Could you check a few things on this model? Use its own coordinates, in mm. Face numbers are marked on the shaded views. A direction names the side the tool comes from. Give positions to 0.01 mm unless a question says otherwise; leave off trailing zeros. Loops run counter-clockwise (first coordinate to the right, second up) from the corner with the lowest first, then second, coordinate; pieces in that order, holes last. Notation, with made-up numbers: (-14.5, 17.25) - (10.5, 17.25) arc R33 ccw to (10.5, 45.25) - close; hole circle Ø10 at (36.5, 72). An arc over 180 degrees is marked (long way). One line per item, written item: value. Start each with the question number.
Q1. I want a section at A-A (x = -18). Please give me the cut outline in (y, z), then the cut area to 3 significant figures.
Q2. If we mould it in two halves opening along Z, with no side actions, what happens to the marked faces 1, 2 and 3? For each: released by +Z, released by -Z, zero draft, split by the parting line, or undercut.
Q3. I want a section at D-D (y = 1). Please give me the cut outline in (x, z), then the cut area to 3 significant figures.
Q4. I want a section at B-B (y = -16.25). Please give me the cut outline in (x, z), then the cut area to 3 significant figures.
Q5. For the marked faces 4, 5, 6, 7 and 8, which set-ups out of +Z, -Z, +X, -X, +Y, -Y let a thin tool reach every point of the face, with its end or its side?
Q6. I want a section at C-C (x = 10.5). Please give me the cut outline in (y, z) (3 decimals), then the cut area to 3 significant figures.
Q7. I'm going to push flat-ended pins straight in: P1, Ø10, axis at x = 8.5, y = -10.5, coming from the -Z side; P2, Ø4, axis at y = -5.5, z = 13.5, coming from the -X side; P3, Ø4.5, axis at y = 13.25, z = 25, coming from the -X side; P4, Ø7.5, axis at x = 1, z = 15, coming from the +Y side. Where does each tip first touch, or does it pass through?
Q8. If I drill on line 1 (Z direction, x = -8, y = 13); line 2 (Z direction, x = -2.5, y = 18.5); line 3 (Y direction, x = -8.85, z = 25), over which ranges is the centre line in solid material (lowest first)? Write a range as from..to.
```python
from build123d import *

# Parameters (mm, degrees)
SKETCH_1_W               = 43
SKETCH_1_H               = 39.5
EXTRUDE_1_DEPTH          = 10
SKETCH_2_W               = 43
SKETCH_2_H               = 13
EXTRUDE_2_DEPTH          = 32
SKETCH_3_R               = 2.75
CUT_EXTRUDE_4_DEPTH      = 58.123222073
CHAMFER_1_SIZE           = 3.5
CUT_EXTRUDE_3_DEPTH      = 44.316422983
CUT_EXTRUDE_3_DEPTH_BACK = 44.316422983
SKETCH_6_R               = 1.3
EXTRUDE_3_DEPTH          = 3
SKETCH_9_W               = 19
SKETCH_9_H               = 13
CUT_EXTRUDE_6_DEPTH      = 11
CUT_EXTRUDE_7_DEPTH      = 54.640586313
CHAMFER_2_SIZE           = 6
CUT_EXTRUDE_START        = -32
SKETCH_12_R              = 5.025
CUT_EXTRUDE_10_DEPTH     = 28.1
EXTRUDE_4_DEPTH          = 10
CHAMFER_5_SIZE           = 10
CUT_EXTRUDE_11_DEPTH     = 50.376740476
CHAMFER_7_SIZE           = 4
SKETCH_15_R              = 1.3
CUT_EXTRUDE_12_DEPTH     = 10
SKETCH_21_W              = 32
SKETCH_21_H              = 4.5
EXTRUDE_7_DEPTH          = 10.5
SKETCH_21_3_R            = 1.3
CUT_EXTRUDE_15_DEPTH     = 6
FILLET_2_R               = 3.5
SKETCH_22_R              = 1.3
EXTRUDE_8_DEPTH          = 1
EXTRUDE_9_DEPTH          = 5
FILLET_3_R               = 3


with BuildPart() as part:
    # 草图1 → 凸台-拉伸1 (new, symmetric)
    with BuildSketch(Plane.XY):
        Rectangle(SKETCH_1_W, SKETCH_1_H)
    extrude(amount=EXTRUDE_1_DEPTH, both=True)

    # 草图2 → 凸台-拉伸2 (add, symmetric)
    with BuildSketch(Plane.XY):
        with Locations((0, 13.25)):
            Rectangle(SKETCH_2_W, SKETCH_2_H)
    extrude(amount=EXTRUDE_2_DEPTH, both=True)

    # 草图3 → 切除-拉伸4 (cut, through all)
    with BuildSketch(Plane.ZY.offset(21.5)):
        with Locations((-25, 13.25)):
            Circle(SKETCH_3_R)
        with Locations((25, 13.25)):
            Circle(SKETCH_3_R)
    extrude(amount=-CUT_EXTRUDE_4_DEPTH, mode=Mode.SUBTRACT)

    # 倒角1
    chamfer_1_edges = [part.edges().sort_by_distance(p)[0] for p in [
        (0, 19.75, 32),
    ]]
    chamfer(chamfer_1_edges, length=CHAMFER_1_SIZE)

    # 草图6 → 切除-拉伸3 (cut, two sides: drawn at the far end of the back side and taken through both)
    with BuildSketch(Plane.XY.offset(-CUT_EXTRUDE_3_DEPTH_BACK)):
        with Locations((-18, -6.25)):
            Circle(SKETCH_6_R)
        with Locations((-18, -16.25)):
            Circle(SKETCH_6_R)
        with Locations((-12, -11.25)):
            Circle(SKETCH_6_R)
    extrude(amount=CUT_EXTRUDE_3_DEPTH + CUT_EXTRUDE_3_DEPTH_BACK, mode=Mode.SUBTRACT)

    # 草图7 → 凸台-拉伸3 (add)
    with BuildSketch(Plane.XY.offset(10)):
        Polygon((-21.5, -2.65), (-12.458578644, -2.65), (-8.4, -6.708578644), (-8.4, -19.75), (21.5, -19.75), (21.5, 6.75), (-21.5, 6.75), align=None)
    extrude_3 = extrude(amount=EXTRUDE_3_DEPTH)

    # 镜向3: 凸台-拉伸3 across plane
    add(extrude_3.mirror(Plane.XY))

    # 草图9 → 切除-拉伸6 (cut)
    with BuildSketch(Plane.ZY.offset(21.5)):
        with Locations((-22.5, 13.25)):
            Rectangle(SKETCH_9_W, SKETCH_9_H)
        with Locations((22.5, 13.25)):
            Rectangle(SKETCH_9_W, SKETCH_9_H)
    extrude(amount=-CUT_EXTRUDE_6_DEPTH, mode=Mode.SUBTRACT)

    # 草图10 → 切除-拉伸7 (cut, through all)
    with BuildSketch(Plane.XY.offset(13)):
        Polygon((-3.4, -19.75), (21.5, 6.75), (21.5, -19.75), align=None)
    extrude(amount=-CUT_EXTRUDE_7_DEPTH, mode=Mode.SUBTRACT)

    # 倒角2
    chamfer_2_edges = [part.edges().sort_by_distance(p)[0] for p in [
        (-16, 19.75, -13),
        (-16, 19.75, 13),
    ]]
    chamfer(chamfer_2_edges, length=CHAMFER_2_SIZE)

    # 草图12 → 切除-拉伸10 (cut)
    with BuildSketch(Plane.ZY.offset(10.5).offset(CUT_EXTRUDE_START)):
        with Locations((25, 13.25)):
            Circle(SKETCH_12_R)
        with Locations((-25, 13.25)):
            Circle(SKETCH_12_R)
    extrude(amount=CUT_EXTRUDE_10_DEPTH, mode=Mode.SUBTRACT)

    # 草图13 → 凸台-拉伸4 (add)
    with BuildSketch(Plane.ZY.offset(21.5)):
        Polygon((-13, -2.65), (-10, -2.65), (-10, 12.507359313), (-5.757359313, 16.75), (5.757359313, 16.75), (10, 12.507359313), (10, -2.65), (13, -2.65), (13, 13.75), (7, 19.75), (-7, 19.75), (-13, 13.75), align=None)
    extrude(amount=EXTRUDE_4_DEPTH)

    # 倒角5
    chamfer_5_edges = [part.edges().sort_by_distance(p)[0] for p in [
        (-31.5, -2.65, 11.5),
        (-31.5, -2.65, -11.5),
    ]]
    chamfer(chamfer_5_edges, length=CHAMFER_5_SIZE)

    # 草图14 → 切除-拉伸11 (cut, through all)
    with BuildSketch(Plane.ZY.offset(10.5)):
        Polygon((-21.5, 19.75), (-19, 17.25), (-9.5, 17.25), (-7, 19.75), align=None)
        Polygon((9.5, 17.25), (7, 19.75), (21.5, 19.75), (19, 17.25), align=None)
    extrude(amount=-CUT_EXTRUDE_11_DEPTH, mode=Mode.SUBTRACT)

    # 倒角7
    chamfer_7_edges = [part.edges().sort_by_distance(p)[0] for p in [
        (5.5, 6.75, 13),
        (5.5, 6.75, -13),
    ]]
    chamfer(chamfer_7_edges, length=CHAMFER_7_SIZE)

    # 草图15 → 切除-拉伸12 (cut)
    with BuildSketch(Plane(origin=(21.5, 0, 0), x_dir=(0, 0, -1), z_dir=(1, 0, 0))):
        with Locations((-15, 13.25)):
            Circle(SKETCH_15_R)
        with Locations((15, 13.25)):
            Circle(SKETCH_15_R)
    extrude(amount=-CUT_EXTRUDE_12_DEPTH, mode=Mode.SUBTRACT)

    # 草图21 → 凸台-拉伸7 (add)
    with BuildSketch(Plane(origin=(0, 0, -32), x_dir=(-1, 0, 0), z_dir=(0, 0, -1))):
        with Locations((-5.5, 22)):
            Rectangle(SKETCH_21_W, SKETCH_21_H)
    extrude(amount=-EXTRUDE_7_DEPTH)

    # 草图21<3> → 切除-拉伸15 (cut)
    with BuildSketch(Plane(origin=(0, 0, -32), x_dir=(-1, 0, 0), z_dir=(0, 0, -1))):
        with Locations((7, 20.75)):
            Circle(SKETCH_21_3_R)
        with Locations((-18, 20.75)):
            Circle(SKETCH_21_3_R)
    extrude(amount=-CUT_EXTRUDE_15_DEPTH, mode=Mode.SUBTRACT)

    # 圆角2
    fillet_2_edges = [part.edges().sort_by_distance(p)[0] for p in [
        (21.5, 24.25, -26.75),
        (-10.5, 24.25, -26.75),
    ]]
    fillet(fillet_2_edges, radius=FILLET_2_R)

    # 草图22 → 凸台-拉伸8 (add)
    with BuildSketch(Plane(origin=(0, 0, -32), x_dir=(-1, 0, 0), z_dir=(0, 0, -1))):
        with BuildLine():
            Line((10.5, 6.75), (10.5, 20.75))
            ThreePointArc((10.5, 20.75), (9.474873734, 23.224873734), (7, 24.25))
            Line((7, 24.25), (-18, 24.25))
            ThreePointArc((-18, 24.25), (-20.474873734, 23.224873734), (-21.5, 20.75))
            Line((-21.5, 20.75), (-21.5, 6.75))
            Line((-21.5, 6.75), (10.5, 6.75))
        make_face()
        with Locations((7, 20.75)):
            Circle(SKETCH_22_R, mode=Mode.SUBTRACT)
        with Locations((-18, 20.75)):
            Circle(SKETCH_22_R, mode=Mode.SUBTRACT)
    extrude(amount=EXTRUDE_8_DEPTH)

    # 草图24 → 凸台-拉伸9 (add)
    with BuildSketch(Plane.XZ.offset(-6.75)):
        Polygon((-10.5, 32), (-4.5, 34), (-3, 34.5), (14, 34.5), (15.5, 34), (21.5, 32), align=None)
    extrude(amount=-EXTRUDE_9_DEPTH)

    # 圆角3
    fillet_3_edges = [part.edges().sort_by_distance(p)[0] for p in [
        (-3, 9.25, 34.5),
        (14, 9.25, 34.5),
    ]]
    fillet(fillet_3_edges, radius=FILLET_3_R)


solid = part.part
```
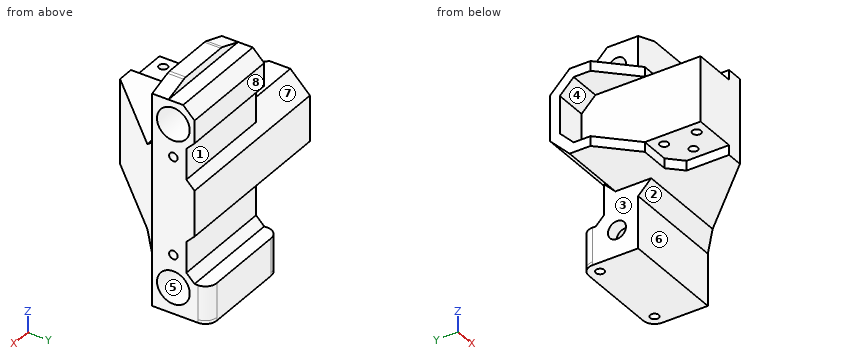
Worked answers:
1. outline: (-19.75, -10) - (-17.55, -10) - (-17.55, 10) - (-19.75, 10) - close; (-14.95, -10) - (-7.55, -10) - (-7.55, 10) - (-14.95, 10) - close; (-4.95, -10) - (-2.65, -10) - (-2.65, -13) - (13.75, -13) - (19.75, -7) - (19.75, 7) - (13.75, 13) - (-2.65, 13) - (-2.65, 10) - (-4.95, 10) - close
1. area: 784 mm²
2. face 1: undercut
2. face 2: released by -Z
2. face 3: zero draft
3. outline: (-25.15, -13) - (16.1, -13) - (16.1, 13) - (-25.15, 13) - (-25.15, 10) - (-21.5, 10) - (-21.5, -10) - (-25.15, -10) - close
3. area: 999 mm²
4. outline: (-21.5, -10) - (-19.3, -10) - (-19.3, 10) - (-21.5, 10) - close; (-16.7, -10) - (-8.4, -10) - (-8.4, -13) - (-0.11, -13) - (-0.11, 13) - (-8.4, 13) - (-8.4, 10) - (-16.7, 10) - close
4. area: 426 mm²
5. face 4: -X, -Y
5. face 5: +X
5. face 6: -Z, +X, -X, -Y
5. face 7: -X, +Y
5. face 8: +Z, +X, -X, +Y
6. outline: (-4.957, -13) - (2.75, -13) - (6.75, -17) - (6.75, -33) - (24.25, -33) - (24.25, -21.5) - (19.75, -21.5) - (17.25, -19) - (17.25, -9.5) - (19.75, -7) - (19.75, 7) - (17.25, 9.5) - (17.25, 19) - (19.75, 21.5) - (19.75, 28.5) - (16.25, 32) - (11.75, 32) - (11.75, 34.5) - (6.75, 34.5) - (6.75, 17) - (2.75, 13) - (-4.957, 13) - close; hole circle Ø10.05 at (13.25, -25); hole circle Ø10.05 at (13.25, 25)
6. area: 1,000 mm²
7. P1: stops at z = -13
7. P2: stops at x = -11.55
7. P3: passes through
7. P4: stops at y = 17.25
8. line 1: z = -33..-27.74, -22.26..22.26, 27.74..32
8. line 2: z = -33..-20.25, -8.25..8.25, 20.25..29.75
8. line 3: y = 6.75..10.5, 16..19.75
